from build123d import *

# Parameters (mm, degrees)
F0_W     = 31.5
F0_H     = 28
F1_DEPTH = 2.5
F0_W_2   = 2.5
F2_DEPTH = 30.5
F4_DEPTH = 2.5
F5_R     = 11.5
F5_R_2   = 2.5
F6_DEPTH = 18.5


with BuildPart() as f1:
    # F0 (on Top) → F1 (new body)
    with BuildSketch(Plane.XY):
        Rectangle(F0_W, F0_H)
    extrude(amount=F1_DEPTH)

    # F0 (on Top) → F2 (join)
    with BuildSketch(Plane.XY):
        with Locations((17, 0)):
            Rectangle(F0_W_2, F0_H)
    extrude(amount=F2_DEPTH)

    # F3 (on face) → F4 (cut)
    with BuildSketch(Plane.YZ.offset(18.25)):
        with BuildLine():
            Line((-11.5, 28), (-10.2, 28))
            ThreePointArc((-10.2, 28), (-12.419239, 28.919239), (-11.5, 26.7))
            Line((-11.5, 26.7), (-11.5, 28))
        make_face()
        with BuildLine():
            Line((-11.5, 5), (-11.5, 6.3))
            ThreePointArc((-11.5, 6.3), (-12.419239, 4.080761), (-10.2, 5))
            Line((-10.2, 5), (-11.5, 5))
        make_face()
        with BuildLine():
            ThreePointArc((-10.2, 5), (-10.580761, 5.919239), (-11.5, 6.3))
            Line((-11.5, 6.3), (-11.5, 5))
            Line((-11.5, 5), (-10.2, 5))
        make_face()
        with BuildLine():
            Line((11.5, 5), (11.5, 6.3))
            ThreePointArc((11.5, 6.3), (10.580761, 5.919239), (10.2, 5))
            Line((10.2, 5), (11.5, 5))
        make_face()
        with BuildLine():
            ThreePointArc((12.8, 5), (12.419239, 5.919239), (11.5, 6.3))
            Line((11.5, 6.3), (11.5, 5))
            Line((11.5, 5), (10.2, 5))
            ThreePointArc((10.2, 5), (11.5, 3.7), (12.8, 5))
        make_face()
        with BuildLine():
            ThreePointArc((11, 16.5), (7.778175, 24.278175), (0, 27.5))
            ThreePointArc((0, 27.5), (-7.778175, 8.721825), (11, 16.5))
        make_face()
        with BuildLine():
            ThreePointArc((-11.5, 26.7), (-10.580761, 27.080761), (-10.2, 28))
            Line((-10.2, 28), (-11.5, 28))
            Line((-11.5, 28), (-11.5, 26.7))
        make_face()
        with BuildLine():
            Line((11.5, 28), (10.2, 28))
            ThreePointArc((10.2, 28), (10.580761, 27.080761), (11.5, 26.7))
            Line((11.5, 26.7), (11.5, 28))
        make_face()
        with BuildLine():
            ThreePointArc((12.8, 28), (11.5, 29.3), (10.2, 28))
            Line((10.2, 28), (11.5, 28))
            Line((11.5, 28), (11.5, 26.7))
            ThreePointArc((11.5, 26.7), (12.419239, 27.080761), (12.8, 28))
        make_face()
    extrude(amount=-F4_DEPTH, mode=Mode.SUBTRACT)

    # F5 (on face) → F6 (join)
    with BuildSketch(Plane(origin=(0, 0, 0), x_dir=(1, 0, 0), z_dir=(0, 0, -1))):
        Circle(F5_R)
        Circle(F5_R_2, mode=Mode.SUBTRACT)
    extrude(amount=F6_DEPTH)


solid = f1.part
Can you work these out from the model? Positions are in its coordinate system, mm. A direction names the side the tool comes from. Coordinates: 2 decimals unless noted, no trailing zeros. Order: outer loops, then holes, each group sorted by start corner. A loop starts at its lowest first (then second) coordinate and runs counter-clockwise, first axis right, second up. Notation, with made-up numbers: (-33, 78) - (-29, 78) arc R11 cw to (-29, 82) - close; hole circle Ø7 at (-19.75, 60). An arc over 180 degrees is marked (long way). Answer as a JSON object with one key per item and string values. Group by question number.
Q1. We'd pull the mould along X, two halves only. Please class faces 1 (the face through (0, 0, 0)), 2 (the face through (-1.5, -11.4, -9.1)), 3 (the face through (0, -3, -18.5)): +X half, -X half, draft (parallel to the pull), parting line (faces both ways), or undercut.
Q2. On a 3-axis mill with a long thin cutter (end or side, diameter ignored), from which of +Z, -Z, +X, -X, +Y, -Y can I reach the whole of each face in a straight line? I mean faces 4 (the face through (9, 14, 2)), 5 (the face through (-0.54, 2.44, -9.12)), 6 (the face through (15.75, -6, 7)). Say none if no direction works.
Q3. Imagine slicing it at C-C (z = -6.5). Please give me the cut outline in (x, y).
Q4. Will these pins go through, and if not, where does the flat tip stop? P1, Ø3, axis at y = -8.5, z = 15.5, coming from the -X side; P2, Ø14, axis at x = -0.5, y = -3.5, coming from the +Z side; P3, Ø3, axis at x = 7, z = -11, coming from the +Y side; P4, Ø8.5, axis at y = 7, z = 12, coming from the -X side.
Q5. I need wall thicknesses on line 1 (Z direction, x = 16.85, y = -11.5); line 2 (Y direction, x = 16.6, z = 5); line 3 (X direction, y = 0, z = -9.25). Which ranges of each line are inside material? Lowest first, please. Write a range as from..to.
Q6. Imagine slicing it at D-D (z = 15). Please give me the cut outline in (x, y), and give its area (3 significant figures).
Q7. Imagine slicing it at B-B (x = -4.5). Please give me the cut outline in (y, z).
Q8. Imagine slicing it at A-A (z = 25). Please give me the cut outline in (x, y), and give its area (3 significant figures).
Determined:
{
 "1": {"face 1": "undercut", "face 2": "parting line", "face 3": "draft"},
 "2": {"face 4": "+Z, -Z, +X, -X, +Y", "face 5": "-Z", "face 6": "+Z, -X, +Y, -Y"},
 "3": {"outline": "circle Ø23 at (0, 0); hole circle Ø5 at (0, 0)"},
 "4": {"P1": "passes through", "P2": "stops at z = 2.5", "P3": "stops at y = 10.1", "P4": "stops at x = 15.75"},
 "5": {"line 1": "z = 0..3.7, 6.3..26.7, 29.3..30.5", "line 2": "y = -14..-12.8, -10.2..10.2, 12.8..14", "line 3": "x = -11.5..-2.5, 2.5..11.5"},
 "6": {"outline": "(15.75, -14) - (18.25, -14) - (18.25, -10.9) - (15.75, -10.9) - close; (15.75, 10.9) - (18.25, 10.9) - (18.25, 14) - (15.75, 14) - close", "area": "15.5 mm2"},
 "7": {"outline": "(-14, 0) - (-10.58, 0) - (-10.58, -18.5) - (10.58, -18.5) - (10.58, 0) - (14, 0) - (14, 2.5) - (-14, 2.5) - close"},
 "8": {"outline": "(15.75, -14) - (18.25, -14) - (18.25, -6.98) - (15.75, -6.98) - close; (15.75, 6.98) - (18.25, 6.98) - (18.25, 14) - (15.75, 14) - close", "area": "35.1 mm2"}
}
